from build123d import *

# Parameters (mm, degrees)
SKETCH1_W           = 1219.2
SKETCH1_H           = 609.6
BOSS_EXTRUDE1_DEPTH = 6.35
SKETCH7_W           = 266.7
SKETCH7_H           = 381
SKETCH7_W_2         = 50.8
BOSS_EXTRUDE2_DEPTH = 25.4


with BuildPart() as part:
    # Sketch1 → Boss-Extrude1 (new body)
    with BuildSketch(Plane(origin=(0, 0, 0), x_dir=(1, 0, 0), z_dir=(0, 1, 0))):
        with Locations((609.6, 304.8)):
            Rectangle(SKETCH1_W, SKETCH1_H)
    extrude(amount=BOSS_EXTRUDE1_DEPTH)

    # Sketch7 → Boss-Extrude2 (add)
    with BuildSketch(Plane(origin=(0, 6.35, 0), x_dir=(1, 0, 0), z_dir=(0, 1, 0))):
        Polygon((1219.2, 609.6), (0, 609.6), (0, 381), (450.85, 381), (501.65, 381), (952.5, 381), (1219.2, 381), align=None)
        with Locations((1085.85, 190.5)):
            Rectangle(SKETCH7_W, SKETCH7_H)
        with Locations((476.25, 190.5)):
            Rectangle(SKETCH7_W_2, SKETCH7_H)
    extrude(amount=BOSS_EXTRUDE2_DEPTH)


solid = part.part
Could you check a few things on this model? Use its own coordinates, in mm. A direction names the side the tool comes from. Give positions to 0.01 mm unless a question says otherwise; leave off trailing zeros. Order: outer loops, then holes, each group sorted by start corner. A loop starts at its lowest first (then second) coordinate and runs counter-clockwise, first axis right, second up. Notation, with made-up numbers: (-17.75, 52.5) - (-5.75, 52.5) arc R14 cw to (-5.75, 56.5) - close; hole circle Ø1 at (66, 69). An arc over 180 degrees is marked (long way). One line per item, written item: value. Start each with the question number.
1. Imagine slicing it at B-B on x = 83.5. List the corners of the cut face in (y, z) for me, plus the area to 3 significant figures.
2. For faces 1 (the face through (724, 6.35, -193)), 2 (the face through (618, 16, -609.6)), 3 (the face through (450.85, 19, -188)), which set-ups out of +Z, -Z, +X, -X, +Y, -Y let a thin tool reach every point of the face, with its end or its side?
3. Imagine slicing it at C-C on y = 22. List the corners of the cut face in (x, z) for me.
4. Thinking about a two-plate mould opening in X: for faces 4 (the face through (501.65, 19, -188)), 5 (the face through (0, 12, -445)), 6 (the face through (601, 0, -309)), which applies, +X half, -X half, draft (parallel to the pull), parting line (faces both ways), or undercut?
5. For P1, Ø12.5, axis at y = 23, z = -111.5, coming from the -X side; P2, Ø12, axis at x = 1057.5, z = -494.5, coming from the -Y side; P3, Ø1, axis at x = 592.5, z = -376.5, coming from the +Y side; P4, Ø6, axis at x = 644.5, y = 13, coming from the +Z side, each with a flat end and sliding along its axis, tell me the tip position at first contact or that it passes through.
6. Imagine slicing it at A-A on z = -119.5. List the corners of the cut face in (x, y) for me.
7. If I drill on probe 1 along X at (y, z) = (7.5, -77.5); probe 2 along Z at (x, y) = (817, 30); probe 3 along Y at (x, z) = (578, -340), over which ranges is the centre line in solid material (lowest first)?
Values:
1. outline: (0, -609.6) - (31.75, -609.6) - (31.75, -381) - (6.35, -381) - (6.35, 0) - (0, 0) - close
1. area: 9,680 mm²
2. face 1: +Z, +Y
2. face 2: -Z, +X, -X, +Y, -Y
2. face 3: +Z, -X, +Y
3. outline: (0, -609.6) - (1219.2, -609.6) - (1219.2, 0) - (952.5, 0) - (952.5, -381) - (501.65, -381) - (501.65, 0) - (450.85, 0) - (450.85, -381) - (0, -381) - close
4. face 4: undercut
4. face 5: -X half
4. face 6: draft
5. P1: x = 450.85
5. P2: y = 0
5. P3: y = 6.35
5. P4: z = -381
6. outline: (0, 0) - (1219.2, 0) - (1219.2, 31.75) - (952.5, 31.75) - (952.5, 6.35) - (501.65, 6.35) - (501.65, 31.75) - (450.85, 31.75) - (450.85, 6.35) - (0, 6.35) - close
7. probe 1: 450.85 to 501.65, 952.5 to 1219.2
7. probe 2: -609.6 to -381
7. probe 3: 0 to 6.35
